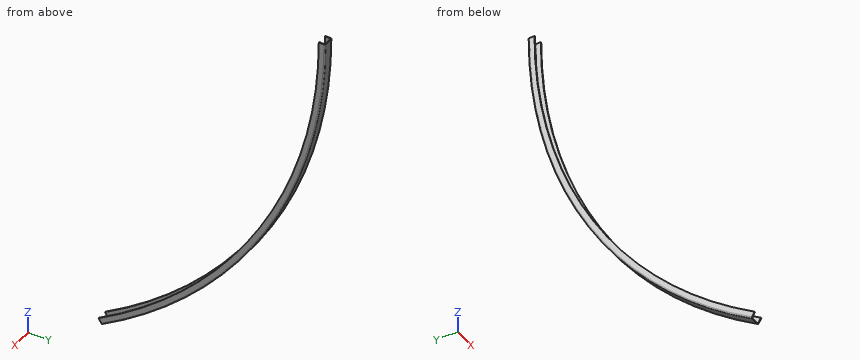
```python
from build123d import *

# Parameters (mm, degrees)
REVOLVE1_ANGLE = 59.5


with BuildPart() as part:
    # Sketch1 → Revolve1 (revolve)
    with BuildSketch(Plane.XY):
        with BuildLine():
            Line((-23.203703704, 37.981481481), (-23.203703704, 54.981481481))
            ThreePointArc((-23.203703704, 54.981481481), (-22.032130828, 57.809908606), (-19.203703704, 58.981481481))
            Line((-19.203703704, 58.981481481), (7.796296296, 58.981481481))
            ThreePointArc((7.796296296, 58.981481481), (10.624723421, 57.809908606), (11.796296296, 54.981481481))
            Line((11.796296296, 54.981481481), (11.796296296, 37.981481481))
            Line((11.796296296, 37.981481481), (9.796296296, 37.981481481))
            Line((9.796296296, 37.981481481), (9.796296296, 54.981481481))
            ThreePointArc((9.796296296, 54.981481481), (9.210509859, 56.395695044), (7.796296296, 56.981481481))
            Line((7.796296296, 56.981481481), (-19.203703704, 56.981481481))
            ThreePointArc((-19.203703704, 56.981481481), (-20.617917266, 56.395695044), (-21.203703704, 54.981481481))
            Line((-21.203703704, 54.981481481), (-21.203703704, 37.981481481))
            Line((-21.203703704, 37.981481481), (-23.203703704, 37.981481481))
        make_face()
    revolve(axis=Axis((14.479414078, -1435.518518519, 0), (-1, 0, 0)), revolution_arc=REVOLVE1_ANGLE)


solid = part.part
```
Here's how the part is built. I have some questions about the finished solid (model axes, mm). Give positions to 0.01 mm unless a question says otherwise; leave off trailing zeros. Order: outer loops, then holes, each group sorted by start corner. A loop starts at its lowest first (then second) coordinate and runs counter-clockwise, first axis right, second up. Notation, with made-up numbers: (-38.75, 31.25) -> (-15.75, 31.25) arc R10 cw to (-15.75, 39.25) -> close; hole circle Ø1 at (-30, 45.5). An arc over 180 degrees is marked (long way). Use CSV: the item, a comma, the result in double quotes. Start each with the question number.
Item 1: I'm going to push flat-ended pins straight in: P1, Ø8, axis at x = -6.5, y = -123, coming from the +Z side; P2, Ø8, axis at x = -6.5, z = -901.5, coming from the +Y side; P3, Ø5, axis at x = -16.5, y = -533.5, coming from the +Z side. Where does each tip first touch, or does it pass through?
Item 2: If I drill on probe 1 along Z at (x, y) = (-16, -335); probe 2 along Y at (x, z) = (-8, -66); probe 3 along Z at (x, y) = (-12.5, -552.5), over which ranges is the centre line in solid material (lowest first)? Write a range as [from, to].
Item 3: Suppose I cut it at A-A (x = -8.5). List the corners of the cut face in (y, z) for me.
Answer block:
1,P1,"stops at z = -703.09"
1,P2,"stops at y = -240.52"
1,P3,"stops at z = -1187.18"
2,probe 1,"z = [-1011.13, -1008.17]"
2,probe 2,"y = [55.52, 57.52]"
2,probe 3,"z = [-1205.74, -1203.26]"
3,outline,"(-678.02, -1285.98) -> (-677, -1287.7) arc R1494.5 ccw to (58.98, 0) -> (56.98, 0) arc R1492.5 cw to start"
